Check sheet for the modelled part. Datum: model origin and axes. Units: mm. A direction names the side the tool comes from. Coordinates: 2 decimals unless noted, no trailing zeros. Loops run counter-clockwise (first coordinate to the right, second up) from the corner with the lowest first, then second, coordinate; pieces in that order, holes last. Notation, with made-up numbers: (56.25, 6) -> (78.25, 6) arc R27 cw to (78.25, 38) -> close; hole circle Ø9 at (16, 74.25). An arc over 180 degrees is marked (long way). Use one line per item in the form item = value.
Autodesk Inventor part; units mm, degrees
ref_plane "YZ Plane" through (0, 0, 0) normal (1, 0, 0) x (0, 1, 0)
ref_plane "XZ Plane" through (0, 0, 0) normal (0, 1, 0) x (-1, 0, 0)
ref_plane "XY Plane" through (0, 0, 0) normal (0, 0, 1) x (1, 0, 0)
sketch "Szkic1" plane through (0, 0, 0) normal (0, 0, 1) x (1, 0, 0)
  line L0 (0, 0) -> (0, 12)
  line L1 (0, 12) -> (-1.5, 12)
  line L2 (-1.5, 12) -> (-1.5, 1.5)
  line L3 (-1.5, 1.5) -> (-12, 1.5)
  line L4 (-12, 1.5) -> (-12, 0)
  line L5 (-12, 0) -> (0, 0)
  dimension "d0" = 12
  dimension "d1" = 1.5
  dimension "d2" = 10.5
  dimension "d3" = 10.5
extrude "Wyciągnięcie proste1" add sketch "Szkic1" along normal mid plane 130
move or copy body "Przesuń bryłę1" bodies to move or copy 1 copy no rotation origin (0, 0, 0) rotation axis (0, 0, 1) rotation angle 90
sketch "Szkic2" plane through (-12, 0, 65) normal (0, 1, 0) x (1, 0, 0)
  line L0 (12, 0) -> (0, 0)
  line L1 (12, 0) -> (12, 130)
  line L2 (0, 130) -> (0, 0) construction
  line L3 (0, 65) -> (5.25, 65) construction
  line L4 (5.25, 79.5) -> (5.25, 50.5) construction
  point P0 (12, 65)
  dimension "d16" = 5.25
  dimension "d17" = 29
hole "Otwór1" at (-6.75, 0, -14.5) at (-6.75, 0, 14.5) direction (0, -1, 0) diameter 3.5 end through all
sketch "Szkic3" plane through (-12, 0, 65) normal (0, 1, 0) x (1, 0, 0)
  line L0 (0, 130) -> (0, 0) construction
  line L1 (12, 0) -> (0, 0) construction
  point P0 (12, 65)
  point P1 (5.25, 5.25)
  dimension "d19" = 5.25
  dimension "d20" = 5.25
hole "Otwór2" at (-6.75, 0, 59.75) direction (0, -1, 0) diameter 3.5 end through all
mirror "Odbij1" about plane through (0, 0, 0) normal (0, 0, 1) of "Otwór2"
sketch "Szkic5" plane through (0, -12, 65) normal (1, 0, 0) x (0, 0, -1)
  line L0 (130, 0) -> (0, 0) construction
  line L1 (65, 0) -> (65, 5.25) construction
  line L2 (30, 5.25) -> (100, 5.25) construction
  point P0 (65, 12)
  dimension "d37" = 5.25
  dimension "d38" = 70
hole "Otwór4" at (0, -6.75, 35) at (0, -6.75, -35) direction (-1, 0, 0) diameter 3.5 end through all
properties part number "bepf_platforma_rama_bok_krotki" material "Aluminium 6061"
(1) Mould release check, pull along Z, two halves, no side actions. Record for faces 1 (the cylindrical face through (-6.08, -0.76, -12.883)), 2 (the flat face through (-1, -3, 65)), 3 (the flat face through (-7, -1.5, -1)): +Z half, -Z half, draft (parallel to the pull), parting line (faces both ways), or undercut.
Established:
face_1 = undercut
face_2 = +Z half
face_3 = draft
(2) Scan lines: line 1 along Z through (x, y) = (-0.45, -6.75); line 2 along Z through (x, y) = (-6.75, -0.7); line 3 along X through (y, z) = (-0.35, -59.75). Record each from-to range of solid material in increasing order.
Established:
line_1 = -65 to -36.75, -33.25 to 33.25, 36.75 to 65
line_2 = -65 to -61.5, -58 to -16.25, -12.75 to 12.75, 16.25 to 58, 61.5 to 65
line_3 = -12 to -8.5, -5 to 0
(3) Section check A-A, the plane z = 35. Record the boundary of the cut face in (x, y), plus the area to 3 significant figures.
Established:
outline = (-12, -1.5) -> (-1.5, -1.5) -> (-1.5, -5) -> (0, -5) -> (0, 0) -> (-12, 0) -> close; (-1.5, -12) -> (0, -12) -> (0, -8.5) -> (-1.5, -8.5) -> close
area = 28.5 mm²
(4) Go/stop test with flat-tipped pins: P1, Ø5, axis at y = -6.5, z = 22.5, coming from the -X side; P2, Ø3, axis at x = -6.75, z = -59.75, coming from the +Y side; P3, Ø4.5, axis at x = -6.75, z = 14.5, coming from the -Y side. Record where each tip stops, or that it passes through.
Established:
P1 = -1.5
P2 = through
P3 = -1.5
(5) Section check B-B, the plane y = -6.75. Record the boundary of the cut face in (x, z), plus the area to 4 significant figures.
Established:
outline = (-1.5, -65) -> (0, -65) -> (0, -36.75) -> (-1.5, -36.75) -> close; (-1.5, -33.25) -> (0, -33.25) -> (0, 33.25) -> (-1.5, 33.25) -> close; (-1.5, 36.75) -> (0, 36.75) -> (0, 65) -> (-1.5, 65) -> close
area = 184.5 mm²
(6) Tool access check on faces 4 (the cylindrical face through (-7.42, -0.76, -61.367)), 5 (the flat face through (-1.5, -7, -1)). Record the directions out of +Z, -Z, +X, -X, +Y, -Y that give a thin tool (end or side, any length) a straight path to the whole face; none if there is none.
Established:
face_4 = +Y, -Y
face_5 = +Z, -Z, -X, -Y
